```python
from build123d import *
from build123d import SkipClean  # not in build123d's __all__

# Parameters (mm, degrees)
F3_DEPTH  = 36
F5_DEPTH  = 20
F7_DEPTH  = 36.001
F10_R     = 10
F11_DEPTH = 7
F12_R     = 10
F12_R_2   = 8
F13_DEPTH = 2
F14_W     = 113.5210208595
F14_H     = 51.0865971446
F15_DEPTH = 38.001
F16_W     = 26.7383140922
F16_H     = 24.3122323528
F17_DEPTH = 36
F18_R     = 2
F20_DEPTH = 5


with BuildPart() as f1:
    # F0 (on Front) → F1 (revolve)
    with BuildSketch(Plane.XZ):
        Polygon((26, -5), (27.5, -5), (27.5, 31), (0, 31), (0, 26), (26, 26), (26, 0), align=None)
    revolve(axis=Axis((0, 0, 28.5), (0, 0, 1)))

    # F2 (on face) → F3 (join, through all)
    with BuildSketch(Plane(origin=(0, 0, -5), x_dir=(1, 0, 0), z_dir=(0, 0, -1))):
        with BuildLine():
            Line((-23.5584379788, 11), (23.5584379788, 11))
            ThreePointArc((23.5584379788, 11), (0, 26), (-23.5584379788, 11))
        make_face()
        with BuildLine():
            Line((23.5584379788, -11), (-23.5584379788, -11))
            ThreePointArc((-23.5584379788, -11), (0, -26), (23.5584379788, -11))
        make_face()
    extrude(amount=-F3_DEPTH)

    # F4 (on Front) → F5 (cut, symmetric)
    with BuildSketch(Plane.XZ):
        with BuildLine():
            Line((4.5, -4.6839690926), (3.5, -1.9364916731))
            ThreePointArc((3.5, -1.9364916731), (3.4457195687, 2.0315060063), (0, 4))
            ThreePointArc((0, 4), (-3.4457195687, 2.0315060063), (-3.5, -1.9364916731))
            Line((-3.5, -1.9364916731), (-4.5, -4.6839690926))
            Line((-4.5, -4.6839690926), (-4.5, -5))
            Line((-4.5, -5), (0, -5))
            Line((0, -5), (4.5, -5))
            Line((4.5, -5), (4.5, -4.6839690926))
        make_face()
    extrude(amount=F5_DEPTH, both=True, mode=Mode.SUBTRACT)

    # F6 (on face) → F7 (cut, through all)
    with BuildSketch(Plane(origin=(0, 0, -5), x_dir=(1, 0, 0), z_dir=(0, 0, -1))):
        with BuildLine():
            Line((24.2332416321, -13), (6.5, -13))
            Line((6.5, -13), (6.5, -22))
            Line((6.5, -22), (-6.5, -22))
            Line((-6.5, -22), (-6.5, -13))
            Line((-6.5, -13), (-24.2332416321, -13))
            ThreePointArc((-24.2332416321, -13), (0, -27.5), (24.2332416321, -13))
        make_face()
        with BuildLine():
            Line((6.5, 22), (6.5, 13))
            Line((6.5, 13), (24.2332416321, 13))
            ThreePointArc((24.2332416321, 13), (0, 27.5), (-24.2332416321, 13))
            Line((-24.2332416321, 13), (-6.5, 13))
            Line((-6.5, 13), (-6.5, 22))
            Line((-6.5, 22), (6.5, 22))
        make_face()
    extrude(amount=-F7_DEPTH, mode=Mode.SUBTRACT)

    # F8 (on Front) → F9 (revolve)
    with BuildSketch(Plane.XZ):
        Polygon((26, -5), (27.5, -5), (27.5, 33), (-8, 33), (-8, 31), (26, 31), align=None)
    revolve(axis=Axis((-8, 0, 32), (0, 0, -1)))

    # F10 (on face) → F11 (cut, through all)
    with BuildSketch(Plane.XY.offset(33)):
        with Locations((-8, 0)):
            Circle(F10_R)
    extrude(amount=-F11_DEPTH, mode=Mode.SUBTRACT)

    # F12 (on face) → F13 (join)
    with BuildSketch(Plane.XY.offset(33)):
        with Locations((-8, 0)):
            Circle(F12_R)
        with Locations((-8, 0)):
            Circle(F12_R_2, mode=Mode.SUBTRACT)
    extrude(amount=-F13_DEPTH)

    # F14 (on face) → F15 (cut, through all)
    with BuildSketch(Plane.XY.offset(33)):
        with Locations((0.0438708812, -25.5432985723)):
            Rectangle(F14_W, F14_H)
    extrude(amount=-F15_DEPTH, mode=Mode.SUBTRACT)

    # F16 (on face) → F17 (cut, through all)
    with BuildSketch(Plane(origin=(0, 0, -5), x_dir=(1, 0, 0), z_dir=(0, 0, -1))):
        with Locations((-19.8691570461, -0.8438838236)):
            Rectangle(F16_W, F16_H)
    extrude(amount=-F17_DEPTH, mode=Mode.SUBTRACT)

    # F18
    f18_edges = [f1.edges().sort_by_distance(p)[0] for p in [
        (-14.627107, 33.347885, 31),
        (-8, 35.5, 33),
        (-6.5, 15.94343, 31),
        (0, 22, 31),
        (6.5, 17.5, 31),
        (14.958278, 13, 31),
    ]]
    fillet(f18_edges, radius=F18_R)

    # F19 (on face) → F20 (cut, through all)
    with BuildSketch(Plane(origin=(0, 0, 26), x_dir=(1, 0, 0), z_dir=(0, 0, -1))):
        with BuildLine():
            ThreePointArc((2, 0), (-0.4171245559, -6.5192024052), (-6.5, -9.8868599666))
            Line((-6.5, -9.8868599666), (-6.5, -11))
            Line((-6.5, -11), (23.5584379788, -11))
            ThreePointArc((23.5584379788, -11), (25.3822712483, -5.6338535902), (26, 0))
            Line((26, 0), (2, 0))
        make_face()
    extrude(amount=-F20_DEPTH, mode=Mode.SUBTRACT)

    # F21: F1 across face


with BuildPart() as f1_1:
    add(f1.part, clean=False)
    with SkipClean():  # cleaning this boolean's faces spoils the solid; the shape is the same uncleaned
        add(f1.part.mirror(Plane(origin=(-36.1785540273, 0, 22.5714053698), x_dir=(1, 0, 0), z_dir=(0, -1, 0))), clean=False)


solid = f1_1.part
```
The model under review builds one solid part; all positions refer to its coordinate system, in mm. A direction names the side the tool comes from. Give positions to 0.01 mm unless a question says otherwise; leave off trailing zeros. Write each loop counter-clockwise with the first axis right and the second up, starting at its lowest first coordinate (ties: lowest second). Pieces come first, ordered by that corner, then holes.
(1) To check wall thickness, follow L1, parallel to Y at x = 0, z = 13.5; L2, parallel to Y at x = 16.5, z = 14; L3, parallel to X at y = 14.25, z = 0. State the ranges of each line that lie inside material, in increasing order.
(2) For P1, Ø13.5, axis at x = 14.5, z = 5, coming from the +Y side; P2, Ø10.5, axis at x = -2, z = 10.5, coming from the -Y side; P3, Ø4.5, axis at y = -16.5, z = 16, coming from the +X side, all flat-tipped, find the tip position at first contact; note any pin that passes through.
(3) The part is to be moulded in two halves that separate along X. For faces 1 (the flat face through (0, -22, 12)), 2 (the flat face through (-6, -13, -5)), say which applies: released by +X, released by -X, zero draft, split by the parting line, or undercut.
(4) Tool access review of faces 3 (the flat face through (-3.993, 15.437, -3.291)), 4 (the cylindrical face through (0, 15, 4)): name each direction out of +Z, -Z, +X, -X, +Y, -Y from which nothing blocks a thin tool from reaching the whole face with its end or side.
(5) Consider section A-A, the plane z = 0. Give the boundary of the cut face in (x, y).
Returned:
1. L1: y = -34.59 to -33.05, -22 to -11, 11 to 22, 33.05 to 34.59
1. L2: y = -25.69 to -23.57, -13 to -11, 11 to 13, 23.57 to 25.69
1. L3: x = -40.51 to -38.87, -6.5 to -4, 4 to 6.5, 22.87 to 24.51
2. P1: stops at y = 31.81
2. P2: stops at y = -35.49
2. P3: stops at x = 24.51
3. face 1: undercut
3. face 2: zero draft
4. face 3: -Z
4. face 4: none
5. outline: circle Ø71 at (-8, 0); hole (-6.5, -22) - (-6.5, -11) - (-4, -11) - (-4, -20) - (4, -20) - (4, -11) - (23.56, -11) arc R26 ccw to (23.56, 11) - (4, 11) - (4, 20) - (-4, 20) - (-4, 11) - (-6.5, 11) - (-6.5, 22) - (6.5, 22) - (6.5, 13) - (23.42, 13) arc R34 ccw (long way) to (23.42, -13) - (6.5, -13) - (6.5, -22) - close
